Answer from the drawing. Dimensions are ordinates in mm from the lowest x, y and z of the part. A direction names the side the tool comes from. Coordinates: 2 decimals unless noted, no trailing zeros. Order: outer loops, then holes, each group sorted by start corner. A loop starts at its lowest first (then second) coordinate and runs counter-clockwise, first axis right, second up. Notation, with made-up numbers: M -7.5,41.5 L 13.5,41.5 A24 cw 13.5,66.5 Z; hole C 47.5,53.25 d7. An arc over 180 degrees is marked long. Use a Markdown table: item, result.
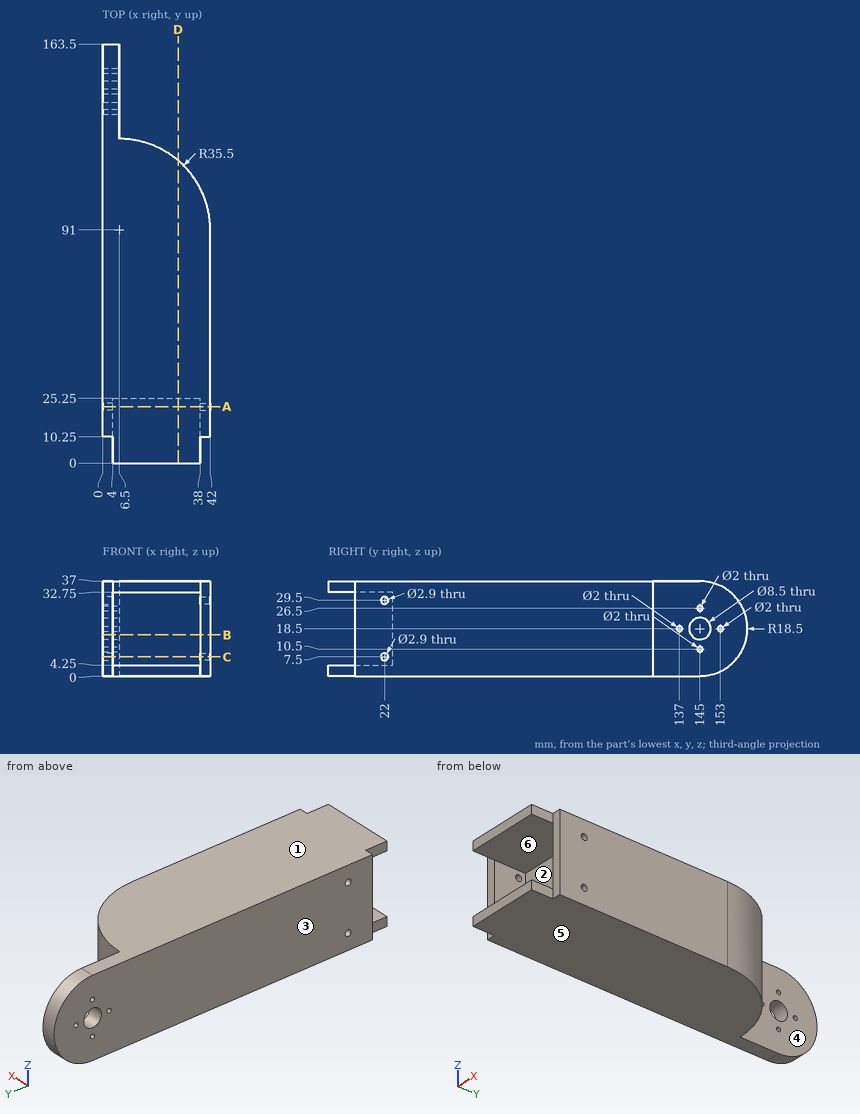
(1) A cutting plane is placed at D-D (x = 29.5). Determine the outline of the cut face in (y, z), then the cut area to 3 significant figures.
Conclusion:
| item | result |
|---|---|
| outline | M 0,0 L 118.04,0 L 118.04,37 L 0,37 L 0,32.75 L 25.25,32.75 L 25.25,4.25 L 0,4.25 Z |
| area | 3,650 mm2 |
(2) Given P1, Ø18.5, axis at y = 151.5, z = 23, coming from the +X side; P2, Ø5, axis at x = 7, z = 30, coming from the -Y side; P3, Ø2, axis at y = 5, z = 3, coming from the -X side; P4, Ø1.2, axis at y = 145, z = 26.5, coming from the -X side, each flat-ended and moving along its own axis, determine where each tip first touches the part or whether it passes through.
Conclusion:
| item | result |
|---|---|
| P1 | x = 6.5 |
| P2 | y = 25.25 |
| P3 | x = 4 |
| P4 | through |
(3) Determine the mould class of the marked faces 1, 2 and 3 for opening direction X: pulls with the +X half, pulls with the -X half, needs draft (parallel to the pull), parting line crosses it, or undercut.
Conclusion:
| item | result |
|---|---|
| face 1 | needs draft |
| face 2 | undercut |
| face 3 | pulls with the -X half |
(4) A cutting plane is placed at C-C (z = 7.5). Determine the outline of the cut face in (x, y).
Conclusion:
| item | result |
|---|---|
| outline | M 0,10.25 L 4,10.25 L 4,20.55 L 0,20.55 Z; M 0,23.45 L 4,23.45 L 4,25.25 L 38,25.25 L 38,23.45 L 42,23.45 L 42,91 A35.5 ccw 6.5,126.5 L 6.5,159.87 L 0,159.87 Z; M 38,10.25 L 42,10.25 L 42,20.55 L 38,20.55 Z |
(5) Which of the six approach directions +Z, -Z, +X, -X, +Y, -Y give full straight-line access (tool end or side, diameter ignored) to the marked faces 4, 5 and 6?
Conclusion:
| item | result |
|---|---|
| face 4 | +Z, -Z, +X, +Y |
| face 5 | -Z, +X, -X, +Y, -Y |
| face 6 | -Y |
(6) A cutting plane is placed at A-A (y = 22). Determine the outline of the cut face in (x, z), then the cut area to 3 significant figures.
Conclusion:
| item | result |
|---|---|
| outline | M 0,0 L 42,0 L 42,6.05 L 38,6.05 L 38,4.25 L 4,4.25 L 4,6.05 L 0,6.05 Z; M 0,8.95 L 4,8.95 L 4,28.05 L 0,28.05 Z; M 0,30.95 L 4,30.95 L 4,32.75 L 38,32.75 L 38,30.95 L 42,30.95 L 42,37 L 0,37 Z; M 38,8.95 L 42,8.95 L 42,28.05 L 38,28.05 Z |
| area | 539 mm2 |
(7) A cutting plane is placed at B-B (z = 16). Determine the outline of the cut face in (x, y), then the cut area to 3 significant figures.
Conclusion:
| item | result |
|---|---|
| outline | M 0,10.25 L 4,10.25 L 4,25.25 L 38,25.25 L 38,10.25 L 42,10.25 L 42,91 A35.5 ccw 6.5,126.5 L 6.5,141.56 L 0,141.56 Z; M 0,148.44 L 6.5,148.44 L 6.5,163.33 L 0,163.33 Z |
| area | 4,300 mm2 |
(8) Straight lines are drawn through the part: L1, parallel to Z at x = 39.7, y = 22; L2, parallel to X at y = 15.5, z = 13; L3, parallel to Z at x = 3.5, y = 145. For each, find the intervals that lie inside material, in ascending order.
Conclusion:
| item | result |
|---|---|
| L1 | 0 to 6.05, 8.95 to 28.05, 30.95 to 37 |
| L2 | 0 to 4, 38 to 42 |
| L3 | 0 to 9.5, 11.5 to 14.25, 22.75 to 25.5, 27.5 to 37 |
